```python
from build123d import *

# Parameters (mm, degrees)
CUT_EXTRUDE1_REACH = 19.854
SKETCH4_R          = 0.477810363


with BuildPart() as part:
    # Sketch2 → Revolve1 (revolve)
    with BuildSketch(Plane.XY, mode=Mode.PRIVATE) as revolve1_sk:
        with BuildLine():
            Line((0, 2.75), (0, 12))
            ThreePointArc((0, 12), (0.146446609, 12.353553391), (0.5, 12.5))
            Line((0.5, 12.5), (4.5, 12.5))
            ThreePointArc((4.5, 12.5), (4.853553391, 12.353553391), (5, 12))
            Line((5, 12), (5, 11))
            ThreePointArc((5, 11), (4.853553391, 10.646446609), (4.5, 10.5))
            Line((4.5, 10.5), (3, 10.5))
            ThreePointArc((3, 10.5), (2.646446609, 10.353553391), (2.5, 10))
            Line((2.5, 10), (2.5, 2.75))
            Line((2.5, 2.75), (0, 2.75))
        make_face()
    revolve(revolve1_sk.sketch.rotate(Axis((0, 0, 0), (1, 0, 0)), 90), axis=Axis((0, 0, 0), (1, 0, 0)))

    # Sketch4 → Cut-Extrude1 (cut, up to next)
    with BuildSketch(Plane(origin=(2.5, 0, 0), x_dir=(0, 0, -1), z_dir=(1, 0, 0)), mode=Mode.PRIVATE) as cut_extrude1_sk1:
        with Locations((8.623339412, -0.147893684)):
            Circle(SKETCH4_R)
    cut_extrude1_tool1 = extrude(cut_extrude1_sk1.sketch, amount=-CUT_EXTRUDE1_REACH, mode=Mode.PRIVATE) & part.part
    add(cut_extrude1_tool1.solids().sort_by_distance((2.5, -0.147894, -8.623339))[0], mode=Mode.SUBTRACT)


solid = part.part
```
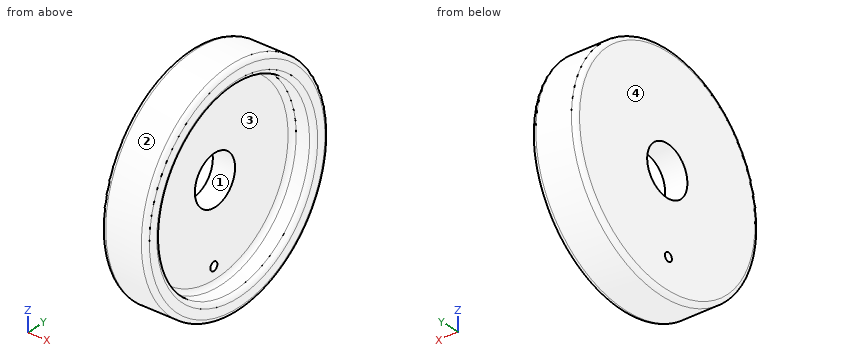
Work out the finished part from the listing and answer in its coordinate system (mm). Face numbers are marked on the shaded views. Give positions to 0.01 mm unless a question says otherwise; leave off trailing zeros. Order: outer loops, then holes, each group sorted by start corner. A loop starts at its lowest first (then second) coordinate and runs counter-clockwise, first axis right, second up. Notation, with made-up numbers: (-18.75, -12) -> (-0.75, -12) arc R8 cw to (-0.75, -6) -> close; hole circle Ø9 at (55, -31.5). An arc over 180 degrees is marked (long way). Answer as CSV lines item,"result". Start each with the question number.
(1) Section C-C, the plane x = 2.05 is taken. Write down the section's boundary in (y, z), plus the area to 3 significant figures.
(2) Section A-A, the plane z = 0 is taken. Write down the section's boundary in (x, y), plus the area to 3 significant figures.
(3) For a pull along Y with two mould halves and no side action, classify the marked faces 1, 2, 3 and 4 as released by +Y, released by -Y, zero draft, split by the parting line, or undercut.
(4) Section B-B, the plane x = 3.3 is taken. Write down the section's boundary in (y, z), plus the area to 3 significant figures.
(5) Consider line 1 along Y through (x, z) = (3.95, 0); line 2 along Y through (x, z) = (1.35, 0); line 3 along Z through (x, y) = (3.1, 4.25). Determine where each line is inside the solid, lowest interval first.
(6) Each of these flat-tipped pins is pushed along its axis until it touches: pin 1 Ø3.5 at (y, z) = (0, 0) entering from +X; pin 2 Ø2 at (x, z) = (4, -4.5) entering from +Y; pin 3 Ø2 at (y, z) = (2, -3) entering from +X; pin 4 Ø1.5 at (x, z) = (2.5, 2.5) entering from +Y. Where does it stop, or does it pass through?
Entries:
1,outline,"circle Ø25 at (0, 0); hole circle Ø5.5 at (0, 0); hole circle Ø0.96 at (-0.15, -8.62)"
1,area,"466 mm²"
2,outline,"(0, -12) arc R0.5 ccw to (0.5, -12.5) -> (4.5, -12.5) arc R0.5 ccw to (5, -12) -> (5, -11) arc R0.5 ccw to (4.5, -10.5) -> (3, -10.5) arc R0.5 cw to (2.5, -10) -> (2.5, -2.75) -> (0, -2.75) -> close; (0, 2.75) -> (2.5, 2.75) -> (2.5, 10) arc R0.5 cw to (3, 10.5) -> (4.5, 10.5) arc R0.5 ccw to (5, 11) -> (5, 12) arc R0.5 ccw to (4.5, 12.5) -> (0.5, 12.5) arc R0.5 ccw to (0, 12) -> close"
2,area,"58.5 mm²"
3,face 1,"undercut"
3,face 2,"split by the parting line"
3,face 3,"undercut"
3,face 4,"zero draft"
4,outline,"circle Ø25 at (0, 0); hole circle Ø21 at (0, 0)"
4,area,"145 mm²"
5,line 1,"-12.5 to -10.5, 10.5 to 12.5"
5,line 2,"-12.5 to -2.75, 2.75 to 12.5"
5,line 3,"-11.76 to -9.6, 9.6 to 11.76"
6,pin 1,"through"
6,pin 2,"y = 12"
6,pin 3,"x = 2.5"
6,pin 4,"y = 12.38"
